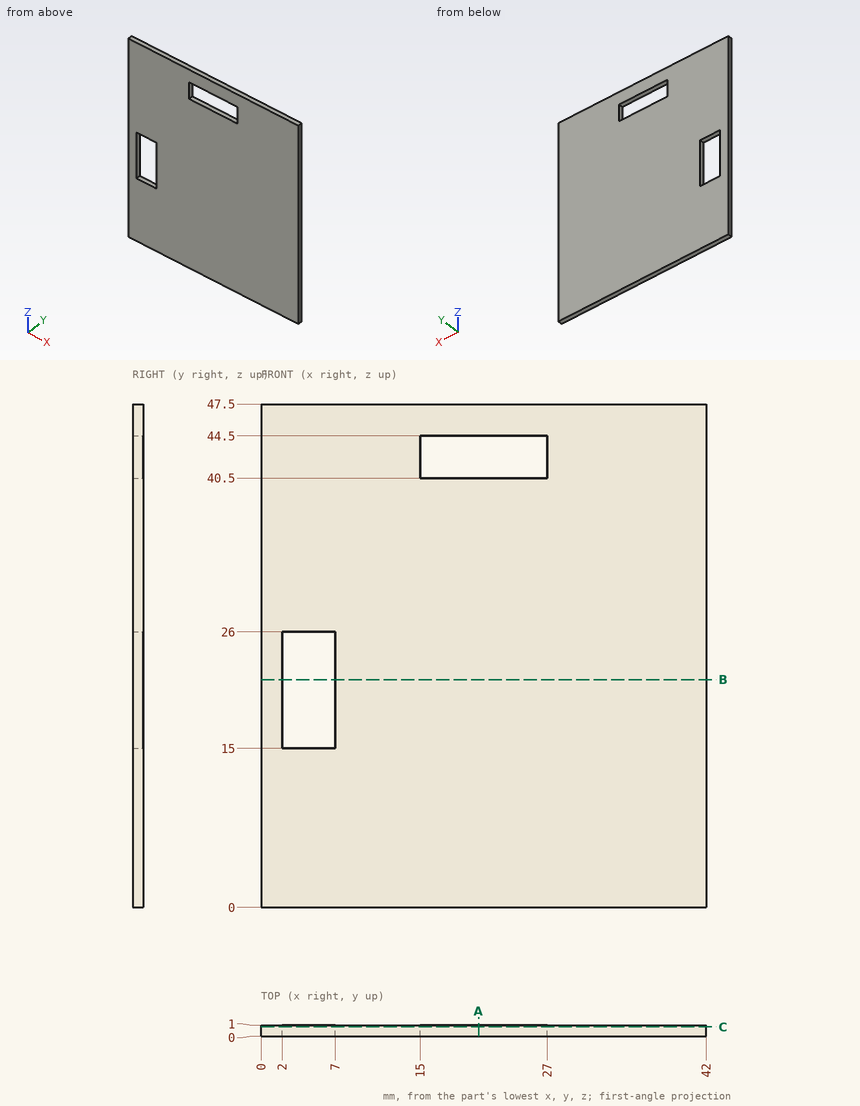
Job drawing, mm, ordinate dimensions from the low corner. One solid piece. Give positions to 0.01 mm unless a question says otherwise; leave off trailing zeros. Order: outer loops, then holes, each group sorted by start corner. A loop starts at its lowest first (then second) coordinate and runs counter-clockwise, first axis right, second up. Notation, with made-up numbers: M 70,20 L 100,20 A19 ccw 100,43 Z; hole C 5,40 d7. An arc over 180 degrees is marked long. Return JSON: item names as keys, results as strings.
Q1. Band-saw the part on B-B (z = 21.5). Give the cut face in (x, y).
Answer list:
{"outline": "M 0,0 L 2,0 L 2,1 L 0,1 Z; M 7,0 L 42,0 L 42,1 L 7,1 Z"}
Q2. Wall check: probe 1 along X at (y, z) = (0.2, 19); probe 2 along Z at (x, y) = (19.5, 0.8); probe 3 along Z at (x, y) = (5, 0.4). Give the ranges that are in metal, low to high. Write a range as from..to.
Answer list:
{"probe 1": "x = 0..2, 7..42", "probe 2": "z = 0..40.5, 44.5..47.5", "probe 3": "z = 0..15, 26..47.5"}
Q3. Band-saw the part on A-A (x = 20.5). Give the cut face in (y, z), then the cut area to 3 significant figures.
Answer list:
{"outline": "M 0,0 L 1,0 L 1,40.5 L 0,40.5 Z; M 0,44.5 L 1,44.5 L 1,47.5 L 0,47.5 Z", "area": "43.5 mm^2"}
Q4. Band-saw the part on C-C (y = 0.85). Give the cut face in (x, z).
Answer list:
{"outline": "M 0,0 L 42,0 L 42,47.5 L 0,47.5 Z; hole M 2,15 L 7,15 L 7,26 L 2,26 Z; hole M 15,40.5 L 27,40.5 L 27,44.5 L 15,44.5 Z"}
